Here's how the part is built. I have some questions about the finished solid (model axes, mm). Face numbers are marked on the shaded views. A direction names the side the tool comes from. Coordinates: 2 decimals unless noted, no trailing zeros. Write each loop counter-clockwise with the first axis right and the second up, starting at its lowest first coordinate (ties: lowest second). Pieces come first, ordered by that corner, then holes.
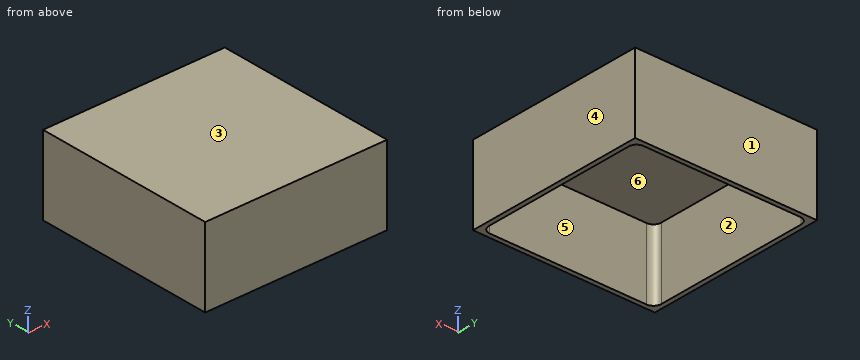
```python
from build123d import *

# Parameters (mm, degrees)
F0_W     = 116
F0_H     = 116
F1_DEPTH = 50
F2_W     = 110
F2_H     = 110
F3_DEPTH = 45
F4_R     = 5


with BuildPart() as f1:
    # F0 (on Top) → F1 (new body)
    with BuildSketch(Plane.XY):
        Rectangle(F0_W, F0_H)
    extrude(amount=F1_DEPTH)

    # F2 (on Top) → F3 (cut)
    with BuildSketch(Plane.XY):
        Rectangle(F2_W, F2_H)
    extrude(amount=F3_DEPTH, mode=Mode.SUBTRACT)

    # F4
    f4_edges = [f1.edges().sort_by_distance(p)[0] for p in [
        (55, 55, 22.5),
        (-55, -55, 22.5),
        (55, -55, 22.5),
        (-55, 55, 22.5),
    ]]
    fillet(f4_edges, radius=F4_R)


solid = f1.part
```
1) We'd pull the mould along X, two halves only. Please class the marked faces 3, 4, 5 and 6: pulls with the +X half, pulls with the -X half, needs draft (parallel to the pull), parting line crosses it, or undercut.
Values follow:
face 3: needs draft
face 4: pulls with the +X half
face 5: undercut
face 6: undercut
2) On a 3-axis mill with a long thin cutter (end or side, diameter ignored), from which of +Z, -Z, +X, -X, +Y, -Y can I reach the whole of each face in a straight line? I mean the marked faces 1 and 2. Say none if no direction works.
Values follow:
face 1: +Z, -Z, +X, -X, +Y
face 2: -Z
3) Imagine slicing it at B-B on x = -35. Please give me the cut outline in (y, z), then the cut area to 3 significant figures.
Values follow:
outline: (-58, 0) - (-55, 0) - (-55, 45) - (55, 45) - (55, 0) - (58, 0) - (58, 50) - (-58, 50) - close
area: 850 mm2
4) I need wall thicknesses on probe 1 along X at (y, z) = (9.5, 25.5); probe 2 along Z at (x, y) = (47, -31). Which ranges of each line are inside material? Lowest first, please.
Values follow:
probe 1: x = -58 to -55, 55 to 58
probe 2: z = 45 to 50
5) Will this pin go through, and if not, where does the flat tip stop? pin 1 (3 mm diameter, centred on x = 38.5, y = -29, fed in from -Z).
Values follow:
pin 1: stops at z = 45
6) Imagine slicing it at A-A on z = 11. Please give me the cut outline in (x, y).
Values follow:
outline: (-58, -58) - (58, -58) - (58, 58) - (-58, 58) - close; hole (-55, -50) arc R5 ccw to (-50, -55) - (50, -55) arc R5 ccw to (55, -50) - (55, 50) arc R5 ccw to (50, 55) - (-50, 55) arc R5 ccw to (-55, 50) - close
